Source: three-view drawing plus pictorial views. Frame: mm from the lowest corner of the part. A direction names the side the tool comes from. Round coordinates to 2 decimals unless told otherwise and drop trailing zeros. Write each loop counter-clockwise with the first axis right and the second up, starting at its lowest first coordinate (ties: lowest second). Pieces come first, ordered by that corner, then holes. Notation, with made-up numbers: (2.25, 19) -> (54.25, 19) arc R23 ccw to (54.25, 45) -> close; hole circle Ø1 at (50, 1.25). An arc over 180 degrees is marked (long way). Put each result on its own line as item: value.
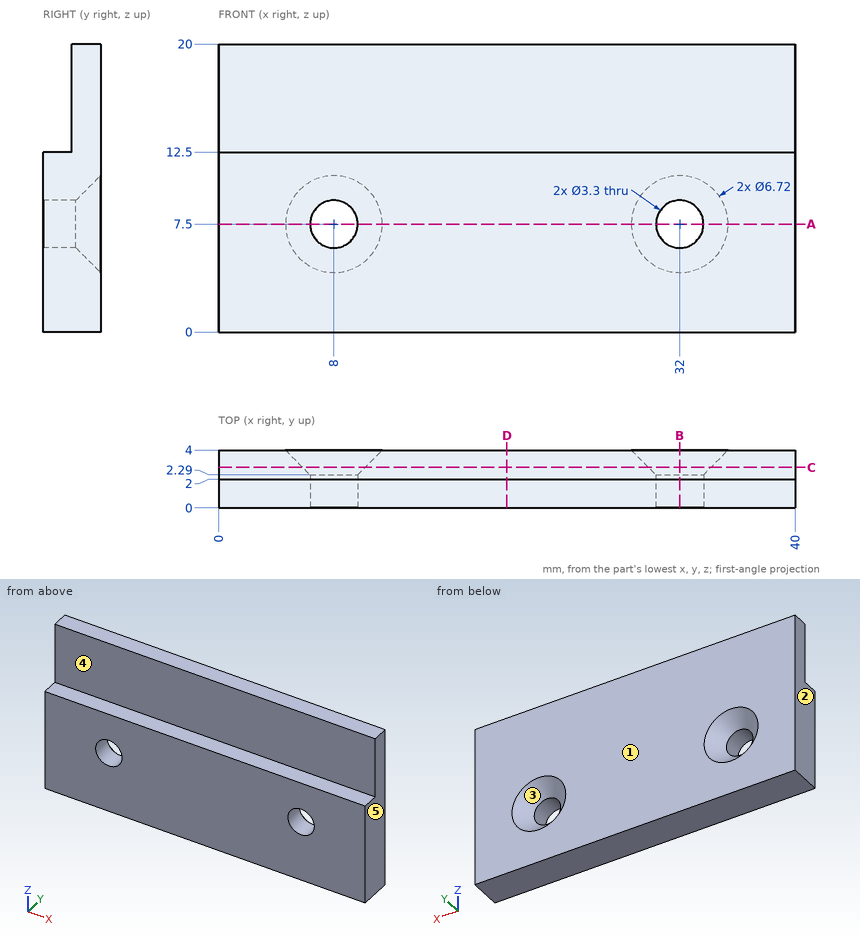
Q1. Cut plane B-B on x = 32. Output: boundary loops of the cut face in (y, z).
Ans:
outline: (0, 0) -> (4, 0) -> (4, 4.14) -> (2.29, 5.85) -> (0, 5.85) -> close; (0, 9.15) -> (2.29, 9.15) -> (4, 10.86) -> (4, 20) -> (2, 20) -> (2, 12.5) -> (0, 12.5) -> close
Q2. Draft query along X for the marked faces 1, 2 and 3. Return one class per face: +X half, -X half, draft (parallel to the pull), parting line (faces both ways), or undercut.
Ans:
face 1: draft
face 2: -X half
face 3: undercut
Q3. Cut plane C-C on y = 2.8. Output: boundary loops of the cut face in (x, z).
Ans:
outline: (0, 0) -> (40, 0) -> (40, 20) -> (0, 20) -> close; hole circle Ø4.32 at (8, 7.5); hole circle Ø4.32 at (32, 7.5)
Q4. Material intervals for line 1 (X direction, y = 1.4, z = 7.5); line 2 (Z direction, x = 8, y = 0.5); line 3 (X direction, y = 3.15, z = 9), sorted ascending. Write a range as [from, to].
Ans:
line 1: x = [0, 6.35], [9.65, 30.35], [33.65, 40]
line 2: z = [0, 5.85], [9.15, 12.5]
line 3: x = [0, 5.99], [10.01, 29.99], [34.01, 40]
Q5. Pin query (flat end, axial travel): pin 1 (1.6 mm diameter, centred on x = 19, y = 0.5, fed in from +Z); pin 2 (2 mm diameter, centred on x = 25.5, z = 17, fed in from -Y); pin 3 (2.5 mm diameter, centred on x = 8, z = 7.5, fed in from -Y). Return the tip coordinate at first contact, or that it passes through.
Ans:
pin 1: stops at z = 12.5
pin 2: stops at y = 2
pin 3: passes through
Q6. Cut plane A-A on z = 7.5. Output: boundary loops of the cut face in (x, y).
Ans:
outline: (0, 0) -> (6.35, 0) -> (6.35, 2.29) -> (4.64, 4) -> (0, 4) -> close; (9.65, 0) -> (30.35, 0) -> (30.35, 2.29) -> (28.64, 4) -> (11.36, 4) -> (9.65, 2.29) -> close; (33.65, 0) -> (40, 0) -> (40, 4) -> (35.36, 4) -> (33.65, 2.29) -> close
Q7. Cut plane D-D on x = 20. Output: boundary loops of the cut face in (y, z), and give its area (3 significant figures).
Ans:
outline: (0, 0) -> (4, 0) -> (4, 20) -> (2, 20) -> (2, 12.5) -> (0, 12.5) -> close
area: 65.0 mm^2
Q8. Reachability of the marked faces 4 and 5 from +Z, -Z, +X, -X, +Y, -Y: full face, straight path, thin tool, end or side. Return the list, or none.
Ans:
face 4: +Z, +X, -X, -Y
face 5: +Z, -Z, +X, +Y, -Y
